Geometry check sheet. Reference: the model listing, model coordinates, mm. Round coordinates to 2 decimals unless told otherwise and drop trailing zeros. Write each loop counter-clockwise with the first axis right and the second up, starting at its lowest first coordinate (ties: lowest second). Pieces come first, ordered by that corner, then holes. Notation, with made-up numbers: (-36.5, -16.5) - (15.5, -16.5) arc R18 ccw to (15.5, 5.5) - close; hole circle Ø4 at (10, 42). An arc over 180 degrees is marked (long way). One line per question, with ' | ' between items. Start each with the question number.
from build123d import *

# Parameters (mm, degrees)
SKETCH1_W             = 273.4
SKETCH1_H             = 263.4
BOSS_EXTRUDE1_DEPTH   = 3
SKETCH2_W             = 43
SKETCH2_H             = 131.64
CUT_EXTRUDE1_DEPTH    = 380.652630703
SKETCH3_W             = 46
SKETCH3_H             = 70
CUT_EXTRUDE2_DEPTH    = 380.652630703
F_4_CLEARANCE_HOLE1_D = 3.2639
CUT_EXTRUDE3_REACH    = 381.653
SKETCH4_R             = 15
F_6_CLEARANCE_HOLE1_D = 3.7973
CUT_EXTRUDE4_REACH    = 381.653


with BuildPart() as part:
    # Sketch1 → Boss-Extrude1 (new body)
    with BuildSketch(Plane.XY):
        with Locations((136.7, -131.7)):
            Rectangle(SKETCH1_W, SKETCH1_H)
    extrude(amount=BOSS_EXTRUDE1_DEPTH)

    # Sketch2 → Cut-Extrude1 (cut, through all)
    with BuildSketch(Plane.XY.offset(3)):
        with Locations((21.5, -65.82)):
            Rectangle(SKETCH2_W, SKETCH2_H)
        with Locations((251.9, -65.82)):
            Rectangle(SKETCH2_W, SKETCH2_H)
    extrude(amount=-CUT_EXTRUDE1_DEPTH, mode=Mode.SUBTRACT)

    # Sketch3 → Cut-Extrude2 (cut, through all)
    with BuildSketch(Plane(origin=(0, 0, 0), x_dir=(-1, 0, 0), z_dir=(0, 0, -1))):
        with Locations((-136.7, -228.4)):
            Rectangle(SKETCH3_W, SKETCH3_H)
    extrude(amount=-CUT_EXTRUDE2_DEPTH, mode=Mode.SUBTRACT)

    # #4 Clearance Hole1 (through all)
    with Locations(Plane(origin=(0, 0, 0), x_dir=(-1, 0, 0), z_dir=(0, 0, -1))):
        with Locations((-267.4, -257.4), (-267.4, -193.4), (-178.4, -193.4), (-178.4, -257.4), (-95, -257.4), (-95, -193.4), (-6, -193.4), (-6, -257.4), (-221.7, -137.5), (-221.7, -182.5), (-51.7, -137.5), (-51.7, -182.5), (-115.45, -17.5), (-157.95, -17.5), (-114.2, -127.5), (-159.2, -127.5), (-61.45, -17.5), (-103.95, -17.5), (-60.2, -127.5), (-105.2, -127.5), (-169.45, -17.5), (-211.95, -17.5), (-168.2, -127.5), (-213.2, -127.5)):
            Hole(F_4_CLEARANCE_HOLE1_D / 2)

    # Sketch4 → Cut-Extrude3 (cut, up to next)
    with BuildSketch(Plane.XY.offset(3), mode=Mode.PRIVATE) as cut_extrude3_sk1:
        with Locations((25.85, -160)):
            Circle(SKETCH4_R)
    cut_extrude3_tool1 = extrude(cut_extrude3_sk1.sketch, amount=-CUT_EXTRUDE3_REACH, mode=Mode.PRIVATE) & part.part
    # Sketch4 → Cut-Extrude3 (cut, up to next)
    with BuildSketch(Plane.XY.offset(3), mode=Mode.PRIVATE) as cut_extrude3_sk2:
        with Locations((247.55, -160)):
            Circle(SKETCH4_R)
    cut_extrude3_tool2 = extrude(cut_extrude3_sk2.sketch, amount=-CUT_EXTRUDE3_REACH, mode=Mode.PRIVATE) & part.part
    # Sketch4 → Cut-Extrude3 (cut, up to next)
    with BuildSketch(Plane.XY.offset(3), mode=Mode.PRIVATE) as cut_extrude3_sk3:
        with BuildLine():
            Line((58, 0), (111.7, 0))
            Line((111.7, 0), (111.7, -2.5))
            ThreePointArc((111.7, -2.5), (110.235533906, -6.035533906), (106.7, -7.5))
            Line((106.7, -7.5), (63, -7.5))
            ThreePointArc((63, -7.5), (59.464466094, -6.035533906), (58, -2.5))
            Line((58, -2.5), (58, 0))
        make_face()
    cut_extrude3_tool3 = extrude(cut_extrude3_sk3.sketch, amount=-CUT_EXTRUDE3_REACH, mode=Mode.PRIVATE) & part.part
    # Sketch4 → Cut-Extrude3 (cut, up to next)
    with BuildSketch(Plane.XY.offset(3), mode=Mode.PRIVATE) as cut_extrude3_sk4:
        with BuildLine():
            Line((43, -48.5), (43, -78.5))
            ThreePointArc((43, -78.5), (58, -63.5), (43, -48.5))
        make_face()
    cut_extrude3_tool4 = extrude(cut_extrude3_sk4.sketch, amount=-CUT_EXTRUDE3_REACH, mode=Mode.PRIVATE) & part.part
    # Sketch4 → Cut-Extrude3 (cut, up to next)
    with BuildSketch(Plane.XY.offset(3), mode=Mode.PRIVATE) as cut_extrude3_sk5:
        with BuildLine():
            Line((230.4, -48.5), (230.4, -78.5))
            ThreePointArc((230.4, -78.5), (215.4, -63.5), (230.4, -48.5))
        make_face()
    cut_extrude3_tool5 = extrude(cut_extrude3_sk5.sketch, amount=-CUT_EXTRUDE3_REACH, mode=Mode.PRIVATE) & part.part
    # Sketch4 → Cut-Extrude3 (cut, up to next)
    with BuildSketch(Plane.XY.offset(3), mode=Mode.PRIVATE) as cut_extrude3_sk6:
        with BuildLine():
            Line((210.4, -7.5), (166.7, -7.5))
            ThreePointArc((166.7, -7.5), (163.164466094, -6.035533906), (161.7, -2.5))
            Line((161.7, -2.5), (161.7, 0))
            Line((161.7, 0), (215.4, 0))
            Line((215.4, 0), (215.4, -2.5))
            ThreePointArc((215.4, -2.5), (213.935533906, -6.035533906), (210.4, -7.5))
        make_face()
    cut_extrude3_tool6 = extrude(cut_extrude3_sk6.sketch, amount=-CUT_EXTRUDE3_REACH, mode=Mode.PRIVATE) & part.part
    add(cut_extrude3_tool1.solids().sort_by_distance((25.85, -160, 3))[0], mode=Mode.SUBTRACT)
    add(cut_extrude3_tool2.solids().sort_by_distance((247.55, -160, 3))[0], mode=Mode.SUBTRACT)
    add(cut_extrude3_tool3.solids().sort_by_distance((84.85, -3.677927, 3))[0], mode=Mode.SUBTRACT)
    add(cut_extrude3_tool4.solids().sort_by_distance((49.366198, -63.5, 3))[0], mode=Mode.SUBTRACT)
    add(cut_extrude3_tool5.solids().sort_by_distance((224.033802, -63.5, 3))[0], mode=Mode.SUBTRACT)
    add(cut_extrude3_tool6.solids().sort_by_distance((188.55, -3.677927, 3))[0], mode=Mode.SUBTRACT)

    # #6 Clearance Hole1 (through all)
    with Locations(Plane.XY.offset(3)):
        with Locations((124.7, -6), (148.7, -6), (9.5, -137.64), (33.5, -137.64), (124.7, -187.4), (148.7, -187.4), (263.9, -137.64), (239.9, -137.64)):
            Hole(F_6_CLEARANCE_HOLE1_D / 2)

    # Sketch9 → Cut-Extrude4 (cut, up to next)
    with BuildSketch(Plane.XY.offset(3), mode=Mode.PRIVATE) as cut_extrude4_sk1:
        with BuildLine():
            Line((72.5, -245.4), (28.5, -245.4))
            ThreePointArc((28.5, -245.4), (8.5, -225.4), (28.5, -205.4))
            Line((28.5, -205.4), (72.5, -205.4))
            ThreePointArc((72.5, -205.4), (92.5, -225.4), (72.5, -245.4))
        make_face()
    cut_extrude4_tool1 = extrude(cut_extrude4_sk1.sketch, amount=-CUT_EXTRUDE4_REACH, mode=Mode.PRIVATE) & part.part
    # Sketch9 → Cut-Extrude4 (cut, up to next)
    with BuildSketch(Plane.XY.offset(3), mode=Mode.PRIVATE) as cut_extrude4_sk2:
        with BuildLine():
            Line((71.7, -145), (201.7, -145))
            ThreePointArc((201.7, -145), (216.7, -160), (201.7, -175))
            Line((201.7, -175), (71.7, -175))
            ThreePointArc((71.7, -175), (56.7, -160), (71.7, -145))
        make_face()
    cut_extrude4_tool2 = extrude(cut_extrude4_sk2.sketch, amount=-CUT_EXTRUDE4_REACH, mode=Mode.PRIVATE) & part.part
    # Sketch9 → Cut-Extrude4 (cut, up to next)
    with BuildSketch(Plane.XY.offset(3), mode=Mode.PRIVATE) as cut_extrude4_sk3:
        with BuildLine():
            Line((154.2, -40), (154.2, -105))
            ThreePointArc((154.2, -105), (136.7, -122.5), (119.2, -105))
            Line((119.2, -105), (119.2, -40))
            ThreePointArc((119.2, -40), (136.7, -22.5), (154.2, -40))
        make_face()
    cut_extrude4_tool3 = extrude(cut_extrude4_sk3.sketch, amount=-CUT_EXTRUDE4_REACH, mode=Mode.PRIVATE) & part.part
    # Sketch9 → Cut-Extrude4 (cut, up to next)
    with BuildSketch(Plane.XY.offset(3), mode=Mode.PRIVATE) as cut_extrude4_sk4:
        with BuildLine():
            Line((208.2, -40), (208.2, -105))
            ThreePointArc((208.2, -105), (190.7, -122.5), (173.2, -105))
            Line((173.2, -105), (173.2, -40))
            ThreePointArc((173.2, -40), (190.7, -22.5), (208.2, -40))
        make_face()
    cut_extrude4_tool4 = extrude(cut_extrude4_sk4.sketch, amount=-CUT_EXTRUDE4_REACH, mode=Mode.PRIVATE) & part.part
    # Sketch9 → Cut-Extrude4 (cut, up to next)
    with BuildSketch(Plane.XY.offset(3), mode=Mode.PRIVATE) as cut_extrude4_sk5:
        with BuildLine():
            Line((100.2, -40), (100.2, -105))
            ThreePointArc((100.2, -105), (82.7, -122.5), (65.2, -105))
            Line((65.2, -105), (65.2, -40))
            ThreePointArc((65.2, -40), (82.7, -22.5), (100.2, -40))
        make_face()
    cut_extrude4_tool5 = extrude(cut_extrude4_sk5.sketch, amount=-CUT_EXTRUDE4_REACH, mode=Mode.PRIVATE) & part.part
    # Sketch9 → Cut-Extrude4 (cut, up to next)
    with BuildSketch(Plane.XY.offset(3), mode=Mode.PRIVATE) as cut_extrude4_sk6:
        with BuildLine():
            Line((200.9, -245.4), (244.9, -245.4))
            ThreePointArc((244.9, -245.4), (264.9, -225.4), (244.9, -205.4))
            Line((244.9, -205.4), (200.9, -205.4))
            ThreePointArc((200.9, -205.4), (180.9, -225.4), (200.9, -245.4))
        make_face()
    cut_extrude4_tool6 = extrude(cut_extrude4_sk6.sketch, amount=-CUT_EXTRUDE4_REACH, mode=Mode.PRIVATE) & part.part
    add(cut_extrude4_tool1.solids().sort_by_distance((50.5, -225.4, 3))[0], mode=Mode.SUBTRACT)
    add(cut_extrude4_tool2.solids().sort_by_distance((136.7, -160, 3))[0], mode=Mode.SUBTRACT)
    add(cut_extrude4_tool3.solids().sort_by_distance((136.7, -72.5, 3))[0], mode=Mode.SUBTRACT)
    add(cut_extrude4_tool4.solids().sort_by_distance((190.7, -72.5, 3))[0], mode=Mode.SUBTRACT)
    add(cut_extrude4_tool5.solids().sort_by_distance((82.7, -72.5, 3))[0], mode=Mode.SUBTRACT)
    add(cut_extrude4_tool6.solids().sort_by_distance((222.9, -225.4, 3))[0], mode=Mode.SUBTRACT)


solid = part.part
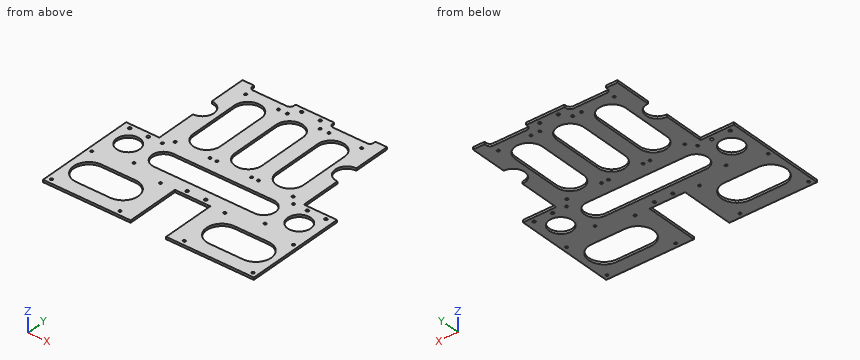
Q1. Section check D-D, the plane z = 2.25. Count the separate pieces of the cut face and the enclosed holes in it, then the cut area to 3 significant figures.
Q2. Go/stop test with flat-tipped pins: P1, Ø0.9, axis at y = -60.5, z = 2, coming from the -X side; P2, Ø1.2, axis at y = -1, z = 2, coming from the -X side. Record where each tip stops, or that it passes through.
Q3. Thickness scan on line 1 (X direction, y = -64, z = 0.25); line 2 (Y direction, x = 6, z = 1.8); line 3 (Y direction, x = 161, z = 0.35). Record the ranges inside material, lowest first.
Q4. Section check B-B, the plane x = 136.7. Record the cut outline in (y, z), then the cut area to 3 significant figures.
Q5. Section check A-A, the plane y = -63.5. Record the cut outline in (x, z), then the cut area to 3 significant figures.
Q6. Section check C-C, the plane x = 187. Record the cut outline in (y, z), then the cut area to 3 significant figures.
Result sheet:
1) separate pieces: 1 | enclosed holes: 40 | area: 33,900 mm²
2) P1: x = 57.6 | P2: x = 43
3) line 1: 57.99 to 65.2, 100.2 to 119.2, 154.2 to 173.2, 208.2 to 215.41 | line 2: -263.4 to -259.03, -255.77 to -195.03, -191.77 to -131.64 | line 3: -263.4 to -175, -145 to 0
4) outline: (-193.4, 0) - (-175, 0) - (-175, 3) - (-193.4, 3) - close; (-145, 0) - (-122.5, 0) - (-122.5, 3) - (-145, 3) - close; (-22.5, 0) - (0, 0) - (0, 3) - (-22.5, 3) - close | area: 190 mm²
5) outline: (58, 0) - (65.2, 0) - (65.2, 3) - (58, 3) - close; (100.2, 0) - (119.2, 0) - (119.2, 3) - (100.2, 3) - close; (154.2, 0) - (173.2, 0) - (173.2, 3) - (154.2, 3) - close; (208.2, 0) - (215.4, 0) - (215.4, 3) - (208.2, 3) - close | area: 157 mm²
6) outline: (-263.4, 0) - (-239.78, 0) - (-239.78, 3) - (-263.4, 3) - close; (-211.02, 0) - (-175, 0) - (-175, 3) - (-211.02, 3) - close; (-145, 0) - (-122.1, 0) - (-122.1, 3) - (-145, 3) - close; (-22.9, 0) - (-7.5, 0) - (-7.5, 3) - (-22.9, 3) - close | area: 294 mm²
